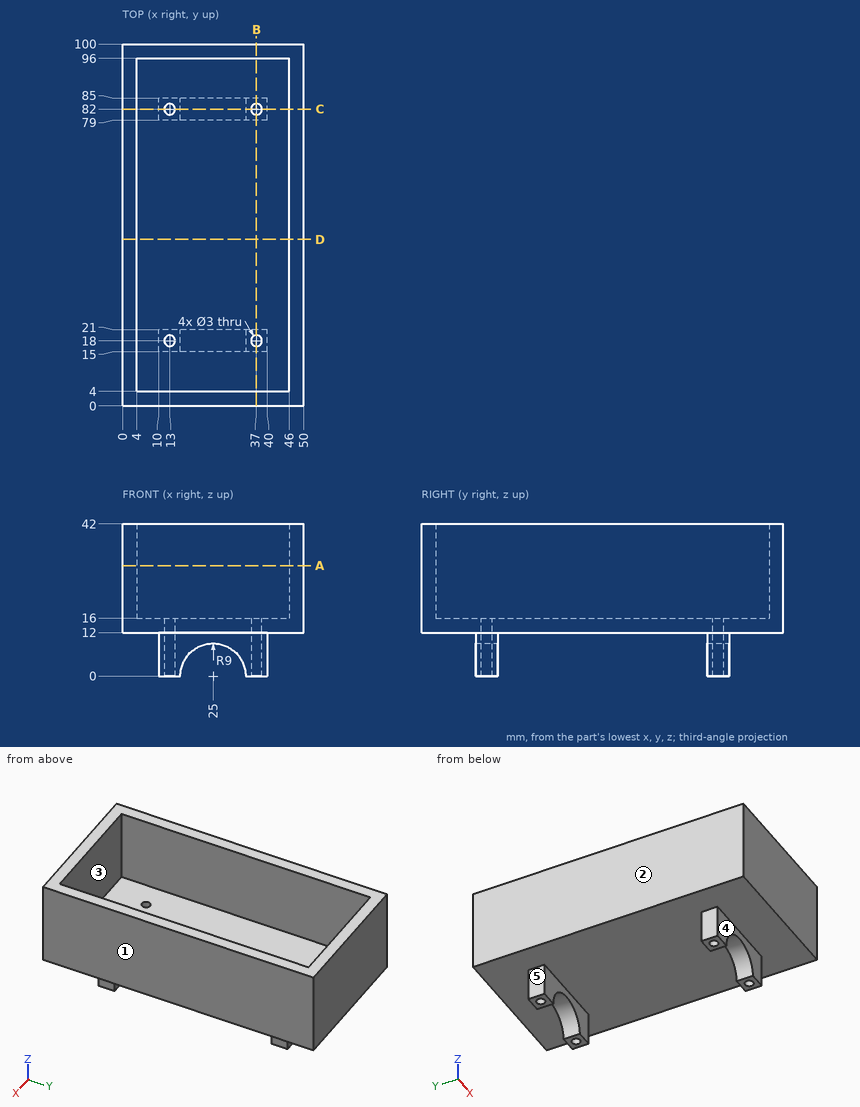
Answer from the drawing. Dimensions are ordinates in mm from the lowest x, y and z of the part. A direction names the side the tool comes from. Round coordinates to 2 decimals unless told otherwise and drop trailing zeros. Loops run counter-clockwise (first coordinate to the right, second up) from the corner with the lowest first, then second, coordinate; pieces in that order, holes last. Notation, with made-up numbers: M 88,51.5 L 92,51.5 A11 cw 92,64.5 Z; hole C -10.75,36 d10. An arc over 180 degrees is marked long. One line per question, with ' | ' between items. Start each with the question number.
(1) A tool of negligible diameter and unlimited length cuts with its end or side. For the marked faces 1, 2, 3, 4 and 5, from which of +Z, -Z, +X, -X, +Y, -Y can it reach the whole face along a straight path? Write none if from no direction.
(2) Find the intervals of material crossed by line 1 (X direction, y = 18, z = 12.75); line 2 (Y direction, x = 37, z = 7); line 3 (Y direction, x = 45.5, z = 17.5), in increasing order.
(3) Flat-ended cylindrical pins translate along their axes: pin 1 Ø3 at (y, z) = (17, 5) entering from -X; pin 2 Ø2 at (y, z) = (82, 6) entering from +X; pin 3 Ø1.5 at (x, z) = (19, 10.5) entering from +Y; pin 4 Ø5 at (y, z) = (88.5, 4.5) entering from +X. Find the tip coordinate at first contact, or state that the pin passes through.
(4) A cutting plane is placed at D-D on y = 46. Write down the section's boundary in (x, z).
(5) A cutting plane is placed at B-B on x = 37. Write down the section's boundary in (y, z).
(6) A cutting plane is placed at A-A on z = 30.5. Write down the section's boundary in (x, y), plus the area to 3 significant figures.
(7) A cutting plane is placed at C-C on y = 82. Write down the section's boundary in (x, z), plus the area to 3 significant figures.
Geometry check:
1) face 1: +Z, -Z, +X, +Y, -Y | face 2: +Z, -Z, -X, +Y, -Y | face 3: +Z | face 4: -Z, +X, -X, -Y | face 5: -Z, -X, +Y, -Y
2) line 1: x = 0 to 11.5, 14.5 to 35.5, 38.5 to 50 | line 2: y = 15 to 16.5, 19.5 to 21, 79 to 80.5, 83.5 to 85 | line 3: y = 0 to 4, 96 to 100
3) pin 1: stops at x = 10 | pin 2: stops at x = 40 | pin 3: stops at y = 85 | pin 4: passes through
4) outline: M 0,12 L 50,12 L 50,42 L 46,42 L 46,16 L 4,16 L 4,42 L 0,42 Z
5) outline: M 0,12 L 15,12 L 15,0 L 16.5,0 L 16.5,16 L 4,16 L 4,42 L 0,42 Z; M 19.5,0 L 21,0 L 21,12 L 79,12 L 79,0 L 80.5,0 L 80.5,16 L 19.5,16 Z; M 83.5,0 L 85,0 L 85,12 L 100,12 L 100,42 L 96,42 L 96,16 L 83.5,16 Z
6) outline: M 0,0 L 50,0 L 50,100 L 0,100 Z; hole M 4,4 L 46,4 L 46,96 L 4,96 Z | area: 1,140 mm²
7) outline: M 0,12 L 10,12 L 10,0 L 11.5,0 L 11.5,16 L 4,16 L 4,42 L 0,42 Z; M 14.5,0 L 16,0 A9 cw 34,0 L 35.5,0 L 35.5,16 L 14.5,16 Z; M 38.5,0 L 40,0 L 40,12 L 50,12 L 50,42 L 46,42 L 46,16 L 38.5,16 Z | area: 545 mm²
